from build123d import *

# Parameters (mm, degrees)
CROQUIS1_R              = 31.5
CROQUIS1_R_2            = 1.5
SALIENTE_EXTRUIR1_DEPTH = 3
CROQUIS4_R              = 2.5
CORTAR_EXTRUIR3_DEPTH   = 3
CROQUIS5_W              = 3
CROQUIS5_H              = 15
SALIENTE_EXTRUIR2_DEPTH = 25
CORTAR_EXTRUIR4_START   = -9
CROQUIS6_R              = 2.7
CORTAR_EXTRUIR4_DEPTH   = 9
CROQUIS7_R              = 3
CORTAR_EXTRUIR5_DEPTH   = 2


with BuildPart() as part:
    # Croquis1 → Saliente-Extruir1 (new body)
    with BuildSketch(Plane.XY):
        with Locations((-43.449193048, 8.207110309)):
            Circle(CROQUIS1_R)
        with Locations((-60.066202406, 24.824119667)):
            Circle(CROQUIS1_R_2, mode=Mode.SUBTRACT)
        with Locations((-26.83218369, 24.824119667)):
            Circle(CROQUIS1_R_2, mode=Mode.SUBTRACT)
        with Locations((-26.83218369, -8.409899049)):
            Circle(CROQUIS1_R_2, mode=Mode.SUBTRACT)
        with Locations((-60.066202406, -8.409899049)):
            Circle(CROQUIS1_R_2, mode=Mode.SUBTRACT)
    extrude(amount=SALIENTE_EXTRUIR1_DEPTH)

    # Croquis4 → Cortar-Extruir3 (cut)
    with BuildSketch(Plane(origin=(0, 0, 0), x_dir=(-1, 0, 0), z_dir=(0, 0, -1))):
        with Locations((43.449193048, 8.207110309)):
            Circle(CROQUIS4_R)
    extrude(amount=-CORTAR_EXTRUIR3_DEPTH, mode=Mode.SUBTRACT)

    # Croquis5 → Saliente-Extruir2 (add)
    with BuildSketch(Plane(origin=(0, 0, 0), x_dir=(-1, 0, 0), z_dir=(0, 0, -1))):
        with Locations((40.449193048, 27.207110309)):
            Rectangle(CROQUIS5_W, CROQUIS5_H)
        with Locations((46.449193048, 27.207110309)):
            Rectangle(CROQUIS5_W, CROQUIS5_H)
    extrude(amount=SALIENTE_EXTRUIR2_DEPTH)

    # Croquis6 → Cortar-Extruir4 (cut)
    with BuildSketch(Plane(origin=(-38.949193048, 0, 0), x_dir=(0, 0, -1), z_dir=(1, 0, 0)).offset(CORTAR_EXTRUIR4_START)):
        with BuildLine():
            Line((25, 34.707110309), (17.5, 34.707110309))
            ThreePointArc((17.5, 34.707110309), (22.803300859, 32.510411168), (25, 27.207110309))
            Line((25, 27.207110309), (25, 34.707110309))
        make_face()
        with BuildLine():
            Line((25, 19.707110309), (25, 27.207110309))
            ThreePointArc((25, 27.207110309), (22.803300859, 21.90380945), (17.5, 19.707110309))
            Line((17.5, 19.707110309), (25, 19.707110309))
        make_face()
        with Locations(Location((17.5, 27.207110309, 0), (0, 0, 90))):
            Circle(CROQUIS6_R)
    extrude(amount=CORTAR_EXTRUIR4_DEPTH, mode=Mode.SUBTRACT)

    # Croquis7 → Cortar-Extruir5 (cut)
    with BuildSketch(Plane(origin=(0, 0, 0), x_dir=(-1, 0, 0), z_dir=(0, 0, -1))):
        with Locations((26.83218369, 24.824119667)):
            Circle(CROQUIS7_R)
        with Locations((60.066202406, 24.824119667)):
            Circle(CROQUIS7_R)
        with Locations((60.066202406, -8.409899049)):
            Circle(CROQUIS7_R)
        with Locations((26.83218369, -8.409899049)):
            Circle(CROQUIS7_R)
    extrude(amount=-CORTAR_EXTRUIR5_DEPTH, mode=Mode.SUBTRACT)


solid = part.part
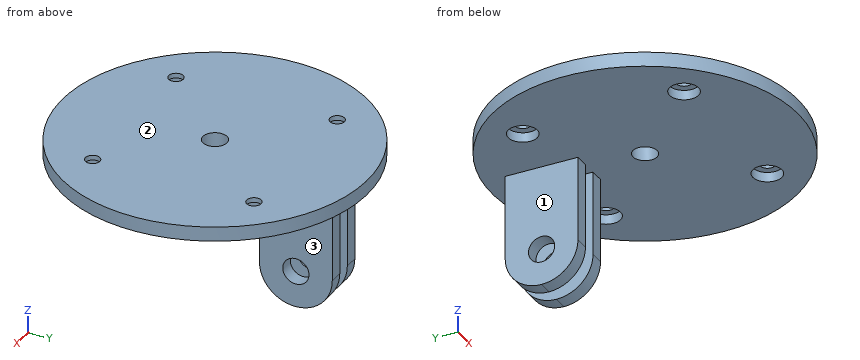
Source: CAD feature listing. Evaluate the final solid. Frame: model axes, mm. Face numbers are marked on the shaded views. A direction names the side the tool comes from. Coordinates: 2 decimals unless noted, no trailing zeros. Loops run counter-clockwise (first coordinate to the right, second up) from the corner with the lowest first, then second, coordinate; pieces in that order, holes last. Notation, with made-up numbers: (-22, -12.5) - (37, -12.5) arc R16 cw to (37, 3.5) - close; hole circle Ø6 at (15, -35.5). An arc over 180 degrees is marked (long way). Return JSON: item names as keys, results as strings.
Q1. Access query for the marked faces 1, 2 and 3. Directions: +Z, -Z, +X, -X, +Y, -Y. A direction counts if a zero-diameter tool reaches every point of the face in a straight line with its end or side. Return the directions, or none.
Results:
{"face 1": "-Z, -X, +Y, -Y", "face 2": "+Z, +X, -X, +Y, -Y", "face 3": "-Z, +X, +Y, -Y"}
Q2. Material intervals for line 1 along Y through (x, z) = (-47.1, -17.5); line 2 along Z through (x, y) = (-34, 36.5); line 3 along Z through (x, y) = (-61, -11), sorted ascending.
Results:
{"line 1": "19.71 to 24.51, 29.91 to 34.71", "line 2": "0 to 3", "line 3": "2 to 3"}
Q3. Section B-B, the plane x = -44. Return loops of the section in (y, z).
Results:
{"outline": "(-23.29, 0) - (5.77, 0) - (5.77, 3) - (-23.29, 3) - close; (10.65, 0) - (39.7, 0) - (39.7, 3) - (10.65, 3) - close"}
Q4. Section D-D, the plane y = 21. Return loops of the section in (x, z).
Results:
{"outline": "(-72.23, 0) - (-47.95, 0) - (-47.95, -21.71) - (-44.95, -21.71) - (-44.95, 0) - (-41.95, 0) - (-41.95, -21.71) - (-38.95, -21.71) - (-38.95, 0) - (-14.66, 0) - (-14.66, 3) - (-72.23, 3) - close"}
Q5. Section A-A, the plane z = -14. Return loops of the section in (x, y), plus the area to 3 significant figures.
Results:
{"outline": "(-47.95, 19.71) - (-44.95, 19.71) - (-44.95, 34.71) - (-47.95, 34.71) - close; (-41.95, 19.71) - (-38.95, 19.71) - (-38.95, 34.71) - (-41.95, 34.71) - close", "area": "90.0 mm2"}
Q6. Contact query for flat-ended pins moving along their axis: P1, Ø1.5, axis at x = -23, y = 27.5, coming from the -Z side; P2, Ø0.9, axis at x = -46, z = -7, coming from the -Y side; P3, Ø2.5, axis at x = -40, z = -9, coming from the +Y side; P4, Ø4.5, axis at y = 27.21, z = -17.5, coming from the +X side. Output: stop coordinate, or through.
Results:
{"P1": "z = 0", "P2": "y = 19.71", "P3": "y = 34.71", "P4": "through"}
Q7. Section C-C, the plane x = -60. Return loops of the section in (y, z), plus the area to 3 significant figures.
Results:
{"outline": "(-18.59, 0) - (-11.41, 0) - (-11.41, 2) - (-9.91, 2) - (-9.91, 3) - (-18.59, 3) - close; (-6.91, 2) - (-5.41, 2) - (-5.41, 0) - (21.82, 0) - (21.82, 2) - (23.33, 2) - (23.33, 3) - (-6.91, 3) - close; (26.32, 2) - (27.82, 2) - (27.82, 0) - (35.01, 0) - (35.01, 3) - (26.32, 3) - close", "area": "131 mm2"}
